```python
from build123d import *

# Parameters (mm, degrees)
F0_R     = 1.25
F1_DEPTH = 10
F2_DEPTH = 15
F3_DEPTH = 8


with BuildPart() as f1:
    # F0 (on Top) → F1 (new body)
    with BuildSketch(Plane.XY):
        Polygon((1.5, 2.598076), (-1.5, 2.598076), (-3, 0), (-1.5, -2.598076), (1.5, -2.598076), (3, 0), align=None)
        Circle(F0_R, mode=Mode.SUBTRACT)
    extrude(amount=F1_DEPTH)

    # F0 (on Top) → F2 (join)
    with BuildSketch(Plane.XY):
        Circle(F0_R)
    extrude(amount=F2_DEPTH)

    # F0 (on Top) → F3 (cut)
    with BuildSketch(Plane.XY):
        Circle(F0_R)
    extrude(amount=F3_DEPTH, mode=Mode.SUBTRACT)


solid = f1.part
```
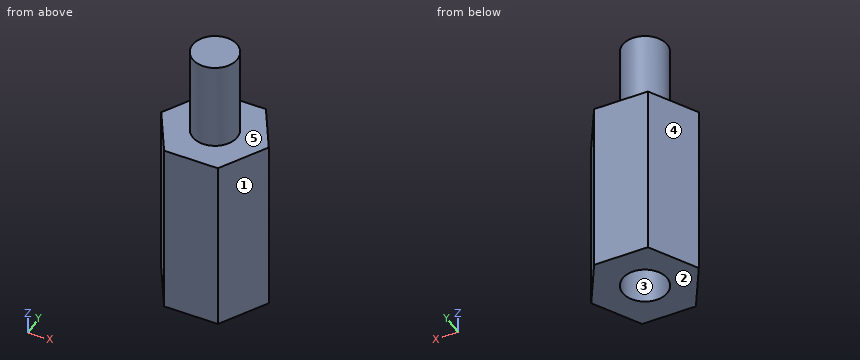
Design review of the part built by this model. Coordinates are the model's own, in mm. Face numbers are marked on the shaded views. A direction names the side the tool comes from. Coordinates: 2 decimals unless noted, no trailing zeros. Write each loop counter-clockwise with the first axis right and the second up, starting at its lowest first coordinate (ties: lowest second). Pieces come first, ordered by that corner, then holes.
1) Machinability: for the marked faces 4 and 5, which of the approach directions +Z, -Z, +X, -X, +Y, -Y give a long, thin tool a straight path to every point of the face, cutting with its end or side? Answer none if there is none.
2) Add section A-A (z = 4.25). Write out the cut boundary in (x, y), plus the area to 3 significant figures.
3) Insertion check: pin 1 (3 mm diameter, centred on y = 0, z = 4.5, fed in from -X); pin 2 (0.8 mm diameter, centred on x = -0.5, y = 0, fed in from -Z). Each pin has a flat end and moves straight along its axis. Give the tip position at first contact, or say it passes through.
4) Add section D-D (y = -1.45). Write out the cut boundary in (x, z).
5) Add section B-B (x = 0). Write out the cut boundary in (y, z).
6) To check wall thickness, follow L1, parallel to Y at x = 0, z = 5.25; L2, parallel to Y at x = 0.9, z = 2.5; L3, parallel to X at y = -0.6, z = 7.75. State the ranges of each line that lie inside material, in increasing order.
7) Add section C-C (y = -0.6). Write out the cut boundary in (x, z).
8) Mouldability with a two-part tool opening along X and no side actions: class the marked faces 1, 2 and 3 as +X half, -X half, draft (parallel to the pull), parting line (faces both ways), or undercut.
Check result:
1. face 4: +Z, -Z, -X, +Y
1. face 5: +Z
2. outline: (-3, 0) - (-1.5, -2.6) - (1.5, -2.6) - (3, 0) - (1.5, 2.6) - (-1.5, 2.6) - close; hole circle Ø2.5 at (0, 0)
2. area: 18.5 mm2
3. pin 1: stops at x = -3
3. pin 2: stops at z = 8
4. outline: (-2.16, 0) - (2.16, 0) - (2.16, 10) - (-2.16, 10) - close
5. outline: (-2.6, 0) - (-1.25, 0) - (-1.25, 8) - (1.25, 8) - (1.25, 0) - (2.6, 0) - (2.6, 10) - (1.25, 10) - (1.25, 15) - (-1.25, 15) - (-1.25, 10) - (-2.6, 10) - close
6. L1: y = -2.6 to -1.25, 1.25 to 2.6
6. L2: y = -2.6 to -0.87, 0.87 to 2.6
6. L3: x = -2.65 to -1.1, 1.1 to 2.65
7. outline: (-2.65, 0) - (-1.1, 0) - (-1.1, 8) - (1.1, 8) - (1.1, 0) - (2.65, 0) - (2.65, 10) - (1.1, 10) - (1.1, 15) - (-1.1, 15) - (-1.1, 10) - (-2.65, 10) - close
8. face 1: +X half
8. face 2: draft
8. face 3: undercut
